from build123d import *

# Parameters (mm, degrees)
F1_DEPTH = 63.5
F2_DEPTH = 25.4


with BuildPart() as f1:
    # F0 (on Front) → F1 (new body, symmetric)
    with BuildSketch(Plane.XZ):
        Polygon((-41.275, 9.525), (-41.275, -9.525), (41.275, -9.525), (41.275, 9.525), (22.225, 9.525), align=None)
    extrude(amount=F1_DEPTH, both=True)

    # F0 (on Front) → F2 (join, symmetric)
    with BuildSketch(Plane.XZ):
        Polygon((-41.275, 9.525), (-41.275, -9.525), (41.275, -9.525), (41.275, 9.525), (22.225, 9.525), align=None)
        with BuildLine():
            add(Edge.make_bspline(
                [(-41.275, 9.525), (-41.2570908666, 43.8246317208), (13.9917880297, 62.3455643654), (57.1499800845, 61.9251837055)],
                knots=[0, 0, 0, 0, 111.5045109268, 111.5045109268, 111.5045109268, 111.5045109268], degree=3))
            Line((-41.275, 9.525), (22.225, 9.525))
            Line((22.225, 9.525), (22.225, 27.0001837055))
            ThreePointArc((22.225, 27.0001837055), (32.4542886259, 51.6958809973), (57.1499800845, 61.9251837055))
        make_face()
        with BuildLine():
            Line((22.225, 9.525), (41.275, 9.525))
            Line((41.275, 9.525), (41.275, 27.0001837055))
            ThreePointArc((41.275, 27.0001837055), (45.9246766481, 38.2255006563), (57.1499909475, 42.8751837055))
            Line((57.1499909475, 42.8751837055), (59.2224501729, 42.8751848873))
            Line((59.2224501729, 42.8751848873), (59.2224501729, 61.9251848873))
            Line((59.2224501729, 61.9251848873), (57.1499800845, 61.9251837055))
            ThreePointArc((57.1499800845, 61.9251837055), (32.4542886259, 51.6958809973), (22.225, 27.0001837055))
            Line((22.225, 27.0001837055), (22.225, 9.525))
        make_face()
        Polygon((84.6224501729, 61.9251993713), (59.2224501729, 61.9251848873), (59.2224501729, 42.8751848873), (84.6224501729, 42.8751993713), align=None)
        Polygon((59.2224501729, 66.675), (59.2224501729, 61.9251848873), (84.6224501729, 61.9251993713), (84.6224501729, 66.675), align=None)
        Polygon((84.6224501729, 42.8751993713), (59.2224501729, 42.8751848873), (59.2224501729, 38.1), (84.6224501729, 38.1), align=None)
        Polygon((84.6224501729, 66.675), (84.6224501729, 61.9251993713), (84.6224501729, 42.8751993713), (84.6224501729, 38.1), (110.0224501729, 38.1), (110.0224501729, 66.675), align=None)
    extrude(amount=F2_DEPTH, both=True)


solid = f1.part
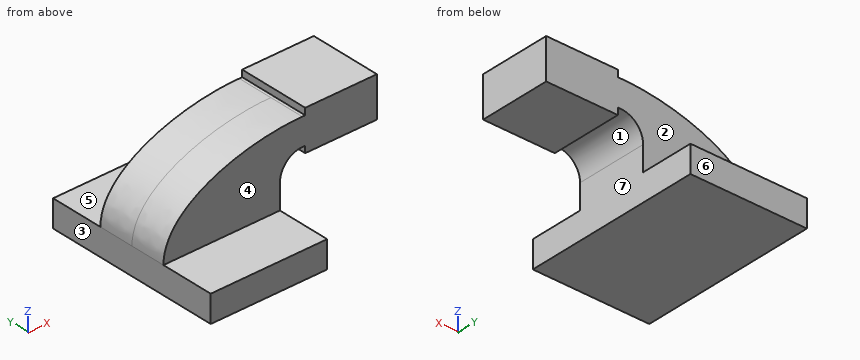
Geometry: final body of the model. Coordinates: model frame, mm. Face numbers are marked on the shaded views. A direction names the side the tool comes from. Round coordinates to 2 decimals unless told otherwise and drop trailing zeros. Loops run counter-clockwise (first coordinate to the right, second up) from the corner with the lowest first, then second, coordinate; pieces in that order, holes last. Notation, with made-up numbers: M 34.25,-36 L 42.25,-36 A29 cw 42.25,-1 Z; hole C -29,27.5 d9. An arc over 180 degrees is marked long. Put each result on its own line as item: value. Start each with the question number.
(1) Contact query for flat-ended pins moving along their axis: pin 1 Ø19 at (x, y) = (1, 43) entering from +Z (3 decimals); pin 2 Ø15 at (x, y) = (76.5, -10.5) entering from -Z; pin 3 Ø6 at (x, z) = (-9, 15.5) entering from +Y. Output: stop coordinate, or through.
(2) Draft query along X for the marked faces 1, 2 and 3. Return one class per face: +X half, -X half, draft (parallel to the pull), parting line (faces both ways), or undercut.
(3) Set-up query: the marked faces 4, 5, 6 and 7. Return all of +Z, -Z, +X, -X, +Y, -Y with unobstructed straight access to the full face (end or side cutting, diameter ignored); none if empty.
(4) Section query A-A (y = -55). Return loops of the section in (x, z) (3 decimals), then the cut area to 3 significant figures.
(5) Material intervals for line 1 along Y through (x, z) = (-11.5, 24); line 2 along X through (y, z) = (-57, 6) (3 decimals); line 3 along Z through (x, y) = (90.5, -22.5) (3 decimals), sorted ascending. Write a range as [from, to].
Findings below:
1. pin 1: stops at z = 9.525
1. pin 2: stops at z = 38.1
1. pin 3: stops at y = 25.4
2. face 1: undercut
2. face 2: draft
2. face 3: -X half
3. face 4: +Z, +X, -X, -Y
3. face 5: +Z, +X, -X, +Y
3. face 6: +Z, -Z, +X, -X, +Y
3. face 7: -Z, +X, +Y, -Y
4. outline: M -41.275,-9.525 L 41.275,-9.525 L 41.275,9.525 L -41.275,9.525 Z
4. area: 1,570 mm2
5. line 1: y = [-25.4, 25.4]
5. line 2: x = [-41.275, 41.275]
5. line 3: z = [38.1, 66.675]
